```python
from build123d import *

# Parameters (mm, degrees)
F0_W     = 20
F0_H     = 20
F0_W_2   = 10
F0_H_2   = 10
F1_DEPTH = 20
F2_W     = 10
F2_H     = 10
F3_DEPTH = 20.001
F4_W     = 10
F4_H     = 10
F5_DEPTH = 20.001


with BuildPart() as f1:
    # F0 (on Top) → F1 (new body)
    with BuildSketch(Plane.XY):
        with Locations((10, 10)):
            Rectangle(F0_W, F0_H)
        with Locations((10, 10)):
            Rectangle(F0_W_2, F0_H_2, mode=Mode.SUBTRACT)
    extrude(amount=F1_DEPTH)

    # F2 (on face) → F3 (cut, through all)
    with BuildSketch(Plane.YZ.offset(20)):
        with Locations((10, 10)):
            Rectangle(F2_W, F2_H)
    extrude(amount=-F3_DEPTH, mode=Mode.SUBTRACT)

    # F4 (on face) → F5 (cut, through all)
    with BuildSketch(Plane(origin=(0, 20, 0), x_dir=(-1, 0, 0), z_dir=(0, 1, 0))):
        with Locations((-10, 10)):
            Rectangle(F4_W, F4_H)
    extrude(amount=-F5_DEPTH, mode=Mode.SUBTRACT)


solid = f1.part
```
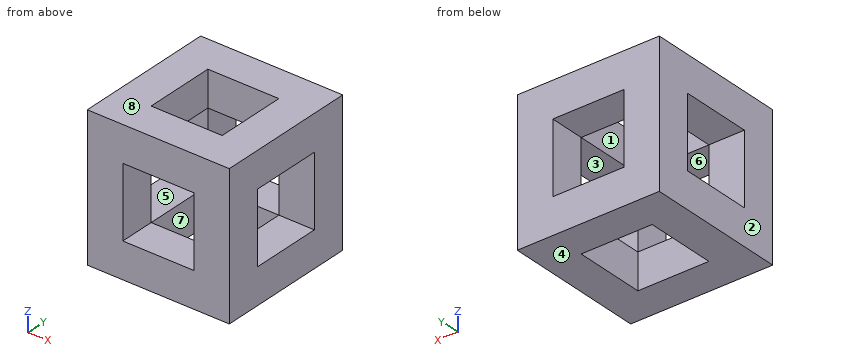
Verification items for the finished model (mm, model axes). Face numbers are marked on the shaded views. A direction names the side the tool comes from. Round coordinates to 2 decimals unless told otherwise and drop trailing zeros. Write each loop counter-clockwise with the first axis right and the second up, starting at its lowest first coordinate (ties: lowest second). Pieces come first, ordered by that corner, then holes. Notation, with made-up numbers: (67, 19.25) - (105, 19.25) arc R19 ccw to (105, 40.25) - close; hole circle Ø9 at (30, 29.5). An arc over 180 degrees is marked (long way). Answer as a JSON object with one key per item and string values. Group by question number.
Q1. Tool access check on the marked faces 4, 5, 6, 7 and 8. Record the directions out of +Z, -Z, +X, -X, +Y, -Y that give a thin tool (end or side, any length) a straight path to the whole face; none if there is none.
Q2. Thickness scan on line 1 (Z direction, x = 2.25, y = 14). Record the ranges inside material, lowest first.
Q3. Section check A-A, the plane y = 9.25. Enter the section's corners in (x, z).
Q4. Mould release check, pull along X, two halves, no side actions. Record for the marked faces 1, 2 and 3: released by +X, released by -X, zero draft, split by the parting line, or undercut.
Q5. Go/stop test with a flat-tipped pin: pin 1 Ø6 at (x, z) = (11.5, 11) entering from +Y. Record where the tip stops, or that it passes through.
Q6. Section check C-C, the plane z = 1.75. Enter the section's corners in (x, y), plus the area to 3 significant figures.
Found:
{
 "1": {"face 4": "-Z, +X, -X, +Y, -Y", "face 5": "+X, -X", "face 6": "+Y, -Y", "face 7": "+Z, -Z", "face 8": "+Z, +X, -X, +Y, -Y"},
 "2": {"line 1": "z = 0 to 5, 15 to 20"},
 "3": {"outline": "(0, 0) - (5, 0) - (5, 5) - (0, 5) - close; (0, 15) - (5, 15) - (5, 20) - (0, 20) - close; (15, 0) - (20, 0) - (20, 5) - (15, 5) - close; (15, 15) - (20, 15) - (20, 20) - (15, 20) - close"},
 "4": {"face 1": "undercut", "face 2": "released by -X", "face 3": "zero draft"},
 "5": {"pin 1": "passes through"},
 "6": {"outline": "(0, 0) - (20, 0) - (20, 20) - (0, 20) - close; hole (5, 5) - (15, 5) - (15, 15) - (5, 15) - close", "area": "300 mm^2"}
}
